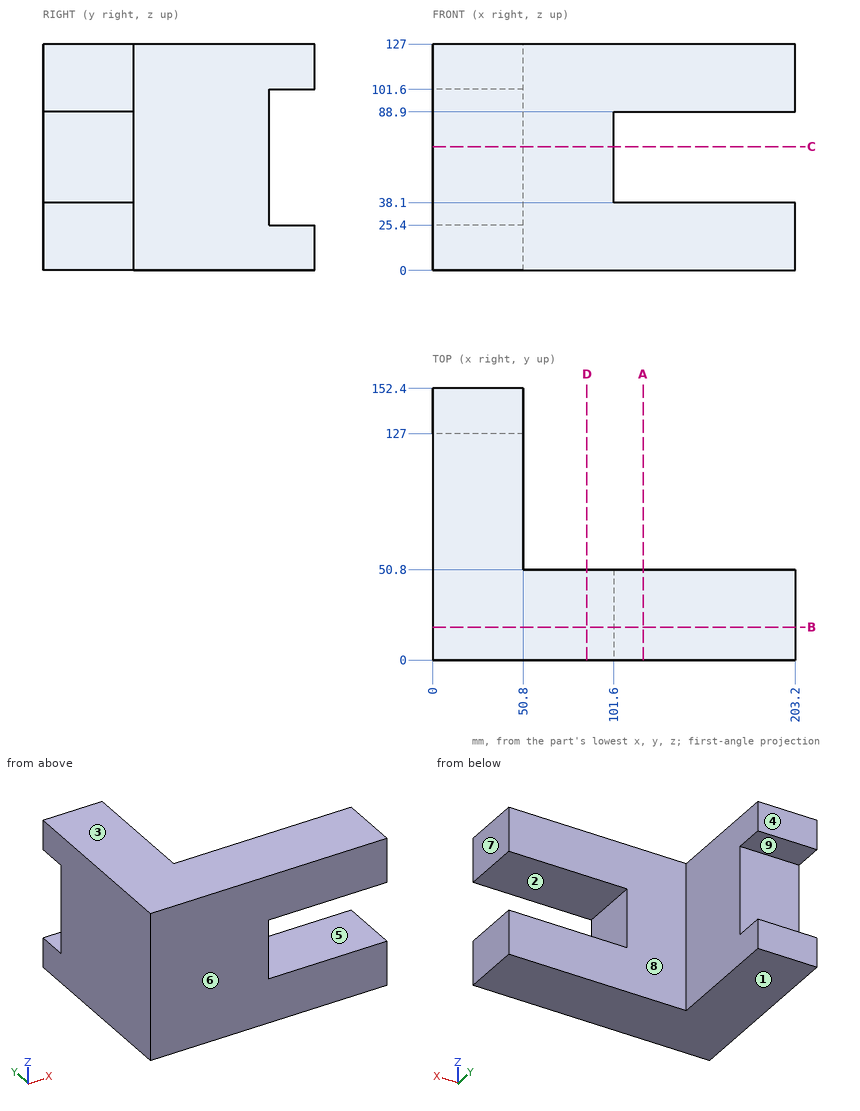
For this review, use the dimensioned drawing (mm, ordinates from the lowest corner) and the shaded views. A direction names the side the tool comes from. Round coordinates to 2 decimals unless told otherwise and drop trailing zeros. Write each loop counter-clockwise with the first axis right and the second up, starting at its lowest first coordinate (ties: lowest second). Pieces come first, ordered by that corner, then holes. Notation, with made-up numbers: (69, -13.75) - (86, -13.75) arc R13 cw to (86, -1.75) - close; hole circle Ø5 at (-24.5, 70). An arc over 180 degrees is marked (long way). Answer as CSV lines item,"result". Start each with the question number.
(1) For the marked faces 5, 6, 7, 8 and 9, list the 3-axis set-ups (+Z, -Z, +X, -X, +Y, -Y) from which the entire face can be reached by the end or side of a thin tool; tool diameter is ignored.
(2) We need section B-B on y = 18.5. State the section outline as (x, z) points.
(3) To check wall thickness, follow line 1 (Z direction, x = 159.5, y = 25); line 2 (X direction, y = 135, z = 19.5). State the ranges of each line that lie inside material, in increasing order.
(4) Draft analysis for pull direction Z (two halves, no side actions). For the marked faces 1, 2, 3 and 4, state which applies: pulls with the +Z half, pulls with the -Z half, needs draft (parallel to the pull), parting line crosses it, or undercut.
(5) We need section A-A on x = 118. State the section outline as (y, z) points.
(6) We need section D-D on x = 86.5. State the section outline as (y, z) points.
(7) We need section C-C on z = 69.5. State the section outline as (x, y) points, plus the area to 3 significant figures.
Worked answers:
1,face 5,"+X, +Y, -Y"
1,face 6,"+Z, -Z, +X, -X, -Y"
1,face 7,"+Z, -Z, +X, +Y, -Y"
1,face 8,"+Z, -Z, +X, +Y"
1,face 9,"+X, -X, +Y"
2,outline,"(0, 0) - (203.2, 0) - (203.2, 38.1) - (101.6, 38.1) - (101.6, 88.9) - (203.2, 88.9) - (203.2, 127) - (0, 127) - close"
3,line 1,"0 to 38.1, 88.9 to 127"
3,line 2,"0 to 50.8"
4,face 1,"pulls with the -Z half"
4,face 2,"undercut"
4,face 3,"pulls with the +Z half"
4,face 4,"needs draft"
5,outline,"(0, 0) - (50.8, 0) - (50.8, 38.1) - (0, 38.1) - close; (0, 88.9) - (50.8, 88.9) - (50.8, 127) - (0, 127) - close"
6,outline,"(0, 0) - (50.8, 0) - (50.8, 127) - (0, 127) - close"
7,outline,"(0, 0) - (101.6, 0) - (101.6, 50.8) - (50.8, 50.8) - (50.8, 127) - (0, 127) - close"
7,area,"9,030 mm²"
